```python
from build123d import *

# Parameters (mm, degrees)
SKETCH1_W           = 26
SKETCH1_H           = 25
BOSS_EXTRUDE1_DEPTH = 1
SKETCH2_R           = 12.5
BOSS_EXTRUDE2_DEPTH = 47
SKETCH3_R           = 6
CUT_EXTRUDE1_DEPTH  = 52.276212809


with BuildPart() as part:
    # Sketch1 → Boss-Extrude1 (new body)
    with BuildSketch(Plane.XY):
        Rectangle(SKETCH1_W, SKETCH1_H)
    extrude(amount=BOSS_EXTRUDE1_DEPTH)

    # Sketch2 → Boss-Extrude2 (add)
    with BuildSketch(Plane.XY.offset(1)):
        with Locations(Location((0, 0, 0), (0, 0, 270))):
            Circle(SKETCH2_R)
    extrude(amount=BOSS_EXTRUDE2_DEPTH)

    # Sketch3 → Cut-Extrude1 (cut, through all)
    with BuildSketch(Plane(origin=(0, 0, 0), x_dir=(-1, 0, 0), z_dir=(0, 0, -1))):
        Circle(SKETCH3_R)
    extrude(amount=-CUT_EXTRUDE1_DEPTH, mode=Mode.SUBTRACT)


solid = part.part
```
Geometry: final body of the model. Coordinates: model frame, mm. A direction names the side the tool comes from. Coordinates: 2 decimals unless noted, no trailing zeros. Order: outer loops, then holes, each group sorted by start corner. A loop starts at its lowest first (then second) coordinate and runs counter-clockwise, first axis right, second up.
Item 1: Contact query for flat-ended pins moving along their axis: P1, Ø3, axis at x = 8, z = 25, coming from the +Y side; P2, Ø4, axis at x = 2.5, z = 36, coming from the +Y side; P3, Ø1.5, axis at x = 4.5, z = 26, coming from the -Y side; P4, Ø11, axis at x = 0, y = 0, coming from the -Z side (3 decimals). Output: stop coordinate, or through.
Answer:
P1: stops at y = 10.68
P2: stops at y = 12.49
P3: stops at y = -11.92
P4: passes through
Item 2: Material intervals for line 1 along Y through (x, z) = (4, 13); line 2 along Y through (x, z) = (-5.5, 12); line 3 along Z through (x, y) = (12.25, -9.5), sorted ascending.
Answer:
line 1: y = -11.84 to -4.47, 4.47 to 11.84
line 2: y = -11.22 to -2.4, 2.4 to 11.22
line 3: z = 0 to 1
Item 3: Draft query along X for faces 1 (the face through (13, -0.2, 0.5)), 2 (the face through (12.7, 1, 1)), 3 (the face through (-13, -0.2, 0.5)), 4 (the face through (6, 0, 24)). Return one class per face: released by +X, released by -X, zero draft, split by the parting line, or undercut.
Answer:
face 1: released by +X
face 2: zero draft
face 3: released by -X
face 4: undercut
Item 4: Section query A-A (y = 0). Output: boundary loops of the cut face in (x, z).
Answer:
outline: (-13, 0) - (-6, 0) - (-6, 48) - (-12.5, 48) - (-12.5, 1) - (-13, 1) - close; (6, 0) - (13, 0) - (13, 1) - (12.5, 1) - (12.5, 48) - (6, 48) - close
Item 5: Access query for faces 5 (the face through (-0.2, -12.5, 0.5)), 6 (the face through (-12.8, -0.9, 1)), 7 (the face through (3.755, -11.923, 24.171)). Directions: +Z, -Z, +X, -X, +Y, -Y. A direction counts if a zero-diameter tool reaches every point of the face in a straight line with its end or side. Return the directions, or none.
Answer:
face 5: +Z, -Z, +X, -X, -Y
face 6: +Z, -X
face 7: +Z
Item 6: Section query D-D (x = 6.5). Output: boundary loops of the cut face in (y, z), then the cut area to 3 significant figures.
Answer:
outline: (-12.5, 0) - (12.5, 0) - (12.5, 1) - (10.68, 1) - (10.68, 48) - (-10.68, 48) - (-10.68, 1) - (-12.5, 1) - close
area: 1,030 mm2
Item 7: Section query B-B (z = 34). Output: boundary loops of the cut face in (x, y), then the cut area to 3 significant figures.
Answer:
outline: circle Ø25 at (0, 0); hole circle Ø12 at (0, 0)
area: 378 mm2
Item 8: Section query C-C (x = -3.5). Output: boundary loops of the cut face in (y, z), then the cut area to 3 significant figures.
Answer:
outline: (-12.5, 0) - (-4.87, 0) - (-4.87, 48) - (-12, 48) - (-12, 1) - (-12.5, 1) - close; (4.87, 0) - (12.5, 0) - (12.5, 1) - (12, 1) - (12, 48) - (4.87, 48) - close
area: 685 mm2
